```python
from build123d import *

# Parameters (mm, degrees)
BOSS_EXTRUDE1_DEPTH   = 9.525
F_4_CLEARANCE_HOLE1_D = 3.2639


with BuildPart() as part:
    # Sketch1 → Boss-Extrude1 (new body)
    with BuildSketch(Plane.XY):
        Polygon((0, 0), (0, -119.888), (24.13, 0), align=None)
    extrude(amount=BOSS_EXTRUDE1_DEPTH)

    # #4 Clearance Hole1 (through all)
    with Locations(Plane.XY.offset(9.525)):
        with Locations((20.6375, -5.842), (4.7625, -5.842)):
            Hole(F_4_CLEARANCE_HOLE1_D / 2)


solid = part.part
```
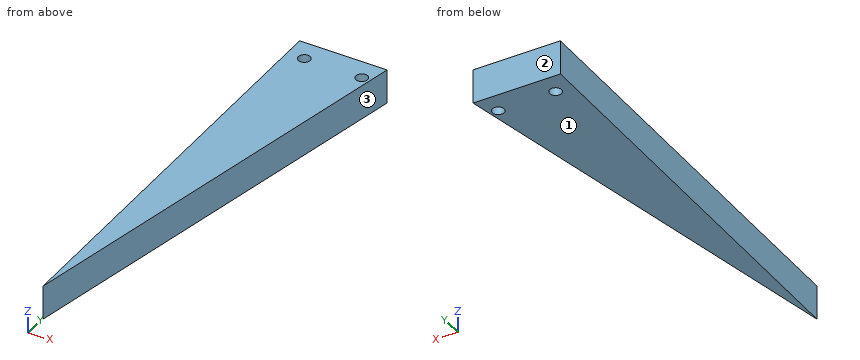
Geometry check sheet. Reference: the model listing, model coordinates, mm. Face numbers are marked on the shaded views. Coordinates: 2 decimals unless noted, no trailing zeros. Order: outer loops, then holes, each group sorted by start corner. A loop starts at its lowest first (then second) coordinate and runs counter-clockwise, first axis right, second up.
Q1. Depth check by flat-ended pin: pin 1 Ø1 at (x, z) = (2.5, 1.5) entering from +Y; pin 2 Ø6 at (x, y) = (11.5, -85) entering from +Z. Enter the tip coordinate at first touch or a pass-through.
Reply:
pin 1: stops at y = 0
pin 2: passes through
Q2. Sectioned sample at B-B on z = 5. Record the cut outline in (x, y).
Reply:
outline: (0, -119.89) - (24.13, 0) - (0, 0) - close; hole circle Ø3.26 at (4.76, -5.84); hole circle Ø3.26 at (20.64, -5.84)
Q3. Sectioned sample at C-C on y = -30.5. Record the cut outline in (x, z) (3 decimals), and give its area (3 significant figures).
Reply:
outline: (0, 0) - (17.991, 0) - (17.991, 9.525) - (0, 9.525) - close
area: 171 mm2
Q4. Sectioned sample at A-A on x = 4.5. Record the cut outline in (y, z) (3 decimals), and give its area (3 significant figures).
Reply:
outline: (-97.53, 0) - (-7.453, 0) - (-7.453, 9.525) - (-97.53, 9.525) - close; (-4.231, 0) - (0, 0) - (0, 9.525) - (-4.231, 9.525) - close
area: 898 mm2
Q5. Sectioned sample at D-D on x = 11.5. Record the cut outline in (y, z) (3 decimals).
Reply:
outline: (-62.751, 0) - (0, 0) - (0, 9.525) - (-62.751, 9.525) - close
Q6. Thickness scan on probe 1 along X at (y, z) = (-82, 5); probe 2 along X at (y, z) = (-101.5, 3.5). Record the ranges inside material, lowest first.
Reply:
probe 1: x = 0 to 7.63
probe 2: x = 0 to 3.7
Q7. Draft check along Y on the marked faces 1, 2 and 3. Enter one of: released by +Y, released by -Y, zero draft, split by the parting line, or undercut.
Reply:
face 1: zero draft
face 2: released by +Y
face 3: released by -Y
